Check sheet for the modelled part. Datum: model origin and axes. Units: mm. A direction names the side the tool comes from. Coordinates: 2 decimals unless noted, no trailing zeros. Loops run counter-clockwise (first coordinate to the right, second up) from the corner with the lowest first, then second, coordinate; pieces in that order, holes last. Notation, with made-up numbers: (13.5, 59) - (44.5, 59) arc R22 cw to (44.5, 88) - close; hole circle Ø10 at (3, 27.25). An arc over 180 degrees is marked (long way). Answer as a JSON object with one key per item and string values. Group by question number.
from build123d import *

# Parameters (mm, degrees)
BOSS_EXTRUDE1_DEPTH = 38
SKETCH2_R           = 9
SKETCH2_R_2         = 4.5
BOSS_EXTRUDE3_DEPTH = 60
SKETCH4_R           = 4.5
CUT_EXTRUDE1_DEPTH  = 61
CUT_EXTRUDE4_DEPTH  = 39
FILLET1_R           = 10
CUT_EXTRUDE5_DEPTH  = 10
SKETCH7_OUTSIDE_W   = 119.562
SKETCH7_OUTSIDE_H   = 85.562
SKETCH7_OUTSIDE_R   = 36
CUT_EXTRUDE6_DEPTH  = 10
FILLET2_R           = 3


with BuildPart() as part:
    # Sketch1 → Boss-Extrude1 (new body)
    with BuildSketch(Plane(origin=(0, 0, 0), x_dir=(0, 0, -1), z_dir=(1, 0, 0))):
        with BuildLine():
            Line((27, 30), (38, 30))
            Line((38, 30), (38, -30))
            Line((38, -30), (-38, -30))
            Line((-38, -30), (-38, 30))
            Line((-38, 30), (-27, 30))
            ThreePointArc((-27, 30), (0, 3), (27, 30))
        make_face()
    extrude(amount=BOSS_EXTRUDE1_DEPTH)

    # Sketch2 → Boss-Extrude3 (add, through all)
    with BuildSketch(Plane(origin=(0, 30, 0), x_dir=(1, 0, 0), z_dir=(0, 1, 0))):
        with Locations((19, -38)):
            Circle(SKETCH2_R)
        with Locations((19, -38)):
            Circle(SKETCH2_R_2, mode=Mode.SUBTRACT)
        with Locations((19, 38)):
            Circle(SKETCH2_R)
        with Locations((19, 38)):
            Circle(SKETCH2_R_2, mode=Mode.SUBTRACT)
    extrude(amount=-BOSS_EXTRUDE3_DEPTH)

    # Sketch4 → Cut-Extrude1 (cut, through all)
    with BuildSketch(Plane(origin=(0, 30, 0), x_dir=(1, 0, 0), z_dir=(0, 1, 0))):
        with Locations((19, -38)):
            Circle(SKETCH4_R)
        with Locations((19, 38)):
            Circle(SKETCH4_R)
    extrude(amount=-CUT_EXTRUDE1_DEPTH, mode=Mode.SUBTRACT)

    # Sketch5 → Cut-Extrude4 (cut, through all)
    with BuildSketch(Plane.ZY):
        Polygon((-47, -30), (-24.579488272, -30), (-47, -10), align=None)
        Polygon((47, -30), (24.579488272, -30), (47, -10), align=None)
    extrude(amount=-CUT_EXTRUDE4_DEPTH, mode=Mode.SUBTRACT)

    # Fillet1
    fillet1_edges = [part.edges().sort_by_distance(p)[0] for p in [
        (19, -30, 24.579488272),
        (19, -30, -24.579488272),
    ]]
    fillet(fillet1_edges, radius=FILLET1_R)

    # Sketch1<3> → Cut-Extrude5 (cut)
    with BuildSketch(Plane(origin=(0, 0, 0), x_dir=(0, 0, -1), z_dir=(1, 0, 0))):
        with BuildLine():
            Line((38, 30), (36, 30))
            ThreePointArc((36, 30), (0, -6), (-36, 30))
            Line((-36, 30), (-38, 30))
            Line((-38, 30), (-38, -30))
            Line((-38, -30), (38, -30))
            Line((38, -30), (38, 30))
        make_face()
    extrude(amount=CUT_EXTRUDE5_DEPTH, mode=Mode.SUBTRACT)

    # Sketch7 outside → Cut-Extrude6 (cut)
    with BuildSketch(Plane(origin=(38, 0, 0), x_dir=(0, 0, -1), z_dir=(1, 0, 0))):
        Rectangle(SKETCH7_OUTSIDE_W, SKETCH7_OUTSIDE_H)
        with Locations((0, 30)):
            Circle(SKETCH7_OUTSIDE_R, mode=Mode.SUBTRACT)
    extrude(amount=-CUT_EXTRUDE6_DEPTH, mode=Mode.SUBTRACT)

    # Fillet2
    fillet2_edges = [part.edges().sort_by_distance(p)[0] for p in [
        (10, -6, 0),
        (28, -6, 0),
    ]]
    fillet(fillet2_edges, radius=FILLET2_R)


solid = part.part
1. Release check for a two-part mould opening along Z. For faces 4 (the face through (38, 2.8, -0.2)), 5 (the face through (22.874, -20.794, -34.9)), 6 (the face through (21.419, 4.296, 34.206)) record: released by +Z, released by -Z, zero draft, split by the parting line, or undercut.
2. Gauge pin test, flat ends, axial feed: pin 1 (15.5 mm diameter, centred on y = -15.5, z = 6, fed in from +X); pin 2 (12 mm diameter, centred on x = 13.5, y = 5.5, fed in from +Z); pin 3 (4 mm diameter, centred on x = 21, z = 7.5, fed in from +Y); pin 4 (10 mm diameter, centred on x = 9.5, z = 27, fed in from -Y). Record the tip position at first contact, or that the pin passes through.
3. Sectioned sample at C-C on y = -4. State how many separate pieces and enclosed holes the cut face has, plus the area to 3 significant figures.
4. Sectioned sample at A-A on x = 19. Record the cut outline in (y, z).
5. Material ranges on line 1 (X direction, y = 2, z = -38); line 2 (Z direction, x = 19, y = 11); line 3 (Z direction, x = 19, y = 10), recorded low to high.
6. Access from +Z, -Z, +X, -X, +Y, -Y to the whole of each face (thin tool, end or side, straight path). Record for faces 1 (the face through (19, 30, -32)), 2 (the face through (34.53, -5.99, -0.79)), 3 (the face through (3.47, -5.99, -0.79)).
7. Sectioned sample at B-B on y = -17. Record the cut outline in (x, z), plus the area to 3 significant figures.
8. Sectioned sample at D-D on x = 2.5. Record the cut outline in (y, z).
Answers follow:
{
 "1": {"face 4": "zero draft", "face 5": "released by -Z", "face 6": "undercut"},
 "2": {"pin 1": "stops at x = 28.12", "pin 2": "stops at z = 47", "pin 3": "stops at y = 4.73", "pin 4": "stops at y = -29.92"},
 "3": {"separate pieces": "1", "enclosed holes": "2", "area": "1,990 mm^2"},
 "4": {"outline": "(-30, -20.77) arc R10 ccw to (-27.46, -27.42) - (-22.04, -33.5) - (30, -33.5) - (30, -27) arc R27 cw to (30, 27) - (30, 33.5) - (-22.04, 33.5) - (-27.46, 27.42) arc R10 ccw to (-30, 20.77) - close; (-14.01, -42.5) - (-10, -47) - (30, -47) - (30, -42.5) - close; (-14.01, 42.5) - (30, 42.5) - (30, 47) - (-10, 47) - close"},
 "5": {"line 1": "x = 10 to 14.5, 23.5 to 28", "line 2": "z = -47 to -42.5, -33.5 to -19.18, 19.18 to 33.5, 42.5 to 47", "line 3": "z = -47 to -42.5, -33.5 to -18.14, 18.14 to 33.5, 42.5 to 47"},
 "6": {"face 1": "+Z, -Z, +X, -X, +Y", "face 2": "+X, -Y", "face 3": "-X, -Y"},
 "7": {"outline": "(10, -38) arc R9 ccw to (10.07, -39.15) - (14.65, -39.15) arc R4.5 cw (long way) to (23.35, -39.15) - (27.93, -39.15) arc R9 ccw to (28, -38) - (28, 38) arc R9 ccw to (27.93, 39.15) - (23.35, 39.15) arc R4.5 cw (long way) to (14.65, 39.15) - (10.07, 39.15) arc R9 ccw to (10, 38) - close", "area": "1,330 mm^2"},
 "8": {"outline": "(30, -36) - (30, -27) arc R27 cw to (30, 27) - (30, 36) arc R36 ccw to start"}
}
